Here's how the part is built. I have some questions about the finished solid (model axes, mm). A direction names the side the tool comes from. Give positions to 0.01 mm unless a question says otherwise; leave off trailing zeros. Write each loop counter-clockwise with the first axis right and the second up, starting at its lowest first coordinate (ties: lowest second). Pieces come first, ordered by that corner, then holes. Notation, with made-up numbers: (-16.5, 9) - (31.5, 9) arc R36 ccw to (31.5, 45) - close; hole circle Ø3 at (-29.75, -21.5). An arc over 180 degrees is marked (long way). One line per item, written item: value. Start each with the question number.
1) We'd pull the mould along X, two halves only. Please class faces 4 (the conical face through (-1.596, -2.692, 11.004)), 5 (the flat face through (3.705, -0.422, -0.196)), 6 (the flat face through (1, -7, -20.32)), 7 (the conical face through (-1.74, 7.835, -2.935)): +X half, -X half, draft (parallel to the pull), parting line (faces both ways), or undercut.
2) On a 3-axis mill with a long thin cutter (end or side, diameter ignored), from which of +Z, -Z, +X, -X, +Y, -Y can I reach the whole of each face in a straight line? I mean faces 1 (the conical face through (-1.35, 2.96, -10.51)), 2 (the conical face through (3.131, -0.037, 11.005)), 3 (the flat face through (0.5, -6.5, 20.32)). Say none if no direction works.
3) Imagine slicing it at D-D on z = -15.5. Write out the boundary of the cut face in (x, y), plus the area to 3 significant figures.
4) Please list where these lines run through material, in increasing order: L1, parallel to Y at x = 0.5, z = 7.5; L2, parallel to X at y = 5, z = 6.5; L3, parallel to X at y = 1.25, z = -5.5. Write a range as [from, to].
5) I'm going to push flat-ended pins straight in: P1, Ø1.5, axis at x = 3.5, z = -6, coming from the +Y side; P2, Ø4, axis at x = -5.5, z = 5.5, coming from the -Y side; P3, Ø4, axis at y = 5.5, z = 12.5, coming from the -X side. Where does each tip first touch, or does it pass through?
6) Imagine slicing it at A-A on z = 0. Write out the boundary of the cut face in (x, y), plus the area to 3 significant figures.
7) Imagine slicing it at B-B on x = -3.25. Count the separate pieces of the cut face and the enclosed holes in it, plus the area to 3 significant figures.
from build123d import *

# Parameters (mm, degrees)
F3_DEPTH = 34.29


with BuildPart() as f1:
    # F0 (on Front) → F1 (revolve)
    with BuildSketch(Plane.XZ):
        Polygon((7.874, 20.32), (6.20684, 20.32), (6.096, 13.97), (6.858, -20.32), (7.874, -20.32), (8.173244, 13.97), align=None)
    revolve(axis=Axis((0, 0, 1.098175), (0, 0, -1)))

    # F2 (on face) → F3 (join)
    with BuildSketch(Plane(origin=(0, 0, -20.32), x_dir=(1, 0, 0), z_dir=(0, 0, -1))):
        with BuildLine():
            Line((1.251042, 2.595763), (-5.939202, 3.429))
            ThreePointArc((-5.939202, 3.429), (-6.12053, 3.093749), (-6.282952, 2.748941))
            Line((-6.282952, 2.748941), (1.2065, 2.089719))
            Line((1.2065, 2.089719), (1.251042, 2.595763))
        make_face()
        with BuildLine():
            ThreePointArc((0, -6.858), (0.381, -6.847408), (0.760823, -6.815667))
            Line((0.760823, -6.815667), (-2.413, 0))
            Line((-2.413, 0), (-2.873518, -0.214447))
            Line((-2.873518, -0.214447), (0, -6.858))
        make_face()
        with BuildLine():
            Line((1.622476, -2.381316), (5.939202, 3.429))
            ThreePointArc((5.939202, 3.429), (5.73953, 3.75366), (5.522129, 4.066726))
            Line((5.522129, 4.066726), (1.2065, -2.089719))
            Line((1.2065, -2.089719), (1.622476, -2.381316))
        make_face()
    extrude(amount=-F3_DEPTH)

    # F4 (on Front) → F5 (revolve, cut)
    with BuildSketch(Plane.XZ):
        Polygon((0, 7.874), (6.096, 13.97), (0, 13.97), align=None)
        Polygon((6.858, -20.32), (6.716924, -13.971567), (0, -7.254644), (0, -20.4724), align=None)
    revolve(axis=Axis((0, 0, 1.098175), (0, 0, -1)), mode=Mode.SUBTRACT)


solid = f1.part
Numbers:
1. face 4: undercut
1. face 5: undercut
1. face 6: draft
1. face 7: parting line
2. face 1: -Z
2. face 2: +Z
2. face 3: +Z, +X, -X, +Y, -Y
3. outline: circle Ø15.83 at (0, 0); hole circle Ø13.5 at (0, 0)
3. area: 53.7 mm^2
4. L1: [-8.1, -6.22], [-2.68, -2.15], [6.22, 8.1]
4. L2: [-6.38, -3.77], [-0.8, -0.08], [3.77, 6.38]
4. L3: [-7.91, -6.41], [-2.43, -1.83], [1.8, 2.46], [6.41, 7.91]
5. P1: y = 7.51
5. P2: y = -7.3
5. P3: x = -7.37
6. outline: circle Ø16.1 at (0, 0); hole (-5.81, -2.71) - (1.21, -2.09) - (1.25, -2.6) - (-5.45, -3.37) arc R6.41 ccw to (5.25, -3.68) - (1.21, 2.09) - (1.62, 2.38) - (5.64, -3.03) arc R6.41 ccw to (0.56, 6.38) - (-2.41, 0) - (-2.87, 0.21) - (-0.2, 6.4) arc R6.41 ccw to start
6. area: 87.2 mm^2
7. separate pieces: 3
7. enclosed holes: 0
7. area: 161 mm^2
